```python
from build123d import *

# Parameters (mm, degrees)
F0_R     = 3.8551712717
F0_R_2   = 1.8170405965
F1_DEPTH = 12.7
F0_W     = 120.9587007761
F0_H     = 68.6061382294
F0_W_2   = 3.2722949982
F0_H_2   = 3.6340802908
F0_W_3   = 15.6750679016
F0_H_3   = 11.3066062331
F0_W_4   = 19.2726254463
F0_H_4   = 13.362351805
F2_DEPTH = 2.54


with BuildPart() as f1:
    # F0 (on Front) → F1 (new body)
    with BuildSketch(Plane.XZ):
        with BuildLine():
            Line((-130.564019084, 68.6061382294), (-120.9587007761, 68.6061382294))
            Line((-120.9587007761, 68.6061382294), (-120.9587007761, 79.2347192764))
            ThreePointArc((-120.9587007761, 79.2347192764), (-128.1642263421, 76.0919600831), (-130.564019084, 68.6061382294))
        make_face()
        with BuildLine():
            Line((120.9587007761, 79.2347192764), (120.9587007761, 68.6061382294))
            Line((120.9587007761, 68.6061382294), (130.564019084, 68.6061382294))
            ThreePointArc((130.564019084, 68.6061382294), (128.1642263421, 76.0919600831), (120.9587007761, 79.2347192764))
        make_face()
        with BuildLine():
            Line((-120.9587007761, -79.2347192764), (-120.9587007761, -68.6061382294))
            Line((-120.9587007761, -68.6061382294), (-130.564019084, -68.6061382294))
            ThreePointArc((-130.564019084, -68.6061382294), (-128.1642263421, -76.0919600831), (-120.9587007761, -79.2347192764))
        make_face()
        with BuildLine():
            Line((130.564019084, -68.6061382294), (120.9587007761, -68.6061382294))
            Line((120.9587007761, -68.6061382294), (120.9587007761, -79.2347192764))
            ThreePointArc((120.9587007761, -79.2347192764), (128.1642263421, -76.0919600831), (130.564019084, -68.6061382294))
        make_face()
        Polygon((-120.9587007761, -68.6061382294), (-120.9587007761, 0), (-120.9587007761, 68.6061382294), (-130.564019084, 68.6061382294), (-130.564019084, -68.6061382294), align=None)
        Polygon((120.9587007761, 68.6061382294), (120.9587007761, 0), (120.9587007761, -68.6061382294), (130.564019084, -68.6061382294), (130.564019084, 68.6061382294), align=None)
        Polygon((0, -68.6061382294), (-120.9587007761, -68.6061382294), (-120.9587007761, -79.2347192764), (120.9587007761, -79.2347192764), (120.9587007761, -68.6061382294), align=None)
        Polygon((-120.9587007761, 68.6061382294), (0, 68.6061382294), (120.9587007761, 68.6061382294), (120.9587007761, 79.2347192764), (-120.9587007761, 79.2347192764), align=None)
        with Locations((0, 74.081890285)):
            Circle(F0_R, mode=Mode.SUBTRACT)
        with Locations((7.9652052373, 73.8249197602)):
            Circle(F0_R_2, mode=Mode.SUBTRACT)
    extrude(amount=F1_DEPTH)

    # F0 (on Front) → F2 (join)
    with BuildSketch(Plane.XZ):
        with Locations((-60.4793503881, 34.3030691147)):
            Rectangle(F0_W, F0_H)
        with Locations((-84.6121534705, 36.4879220724)):
            Rectangle(F0_W_2, F0_H_2, mode=Mode.SUBTRACT)
        with Locations((-86.2483009696, 48.9245094359)):
            Rectangle(F0_W_3, F0_H_3, mode=Mode.SUBTRACT)
        with Locations((60.4793503881, 34.3030691147)):
            Rectangle(F0_W, F0_H)
        with Locations((71.5301930904, 45.069983229)):
            Rectangle(F0_W_4, F0_H_4, mode=Mode.SUBTRACT)
        Polygon((120.9587007761, 0), (0, 0), (0, -17.8872328252), (23.6056204885, -17.8872328252), (50.5872815847, -17.8872328252), (50.5872815847, -26.6241524369), (74.228361249, -26.6241524369), (74.228361249, -47.9525141418), (74.228361249, -55.1476255059), (62.4078214169, -55.1476255059), (62.4078214169, -47.9525141418), (50.5872815847, -47.9525141418), (50.5872815847, -44.3549603224), (20.5219965428, -44.3549603224), (0, -44.3549603224), (0, -68.6061382294), (120.9587007761, -68.6061382294), align=None)
        Polygon((0, -17.8872328252), (0, 0), (-120.9587007761, 0), (-120.9587007761, -68.6061382294), (0, -68.6061382294), (0, -44.3549603224), (-2.8621072415, -44.3549603224), (-2.8621072415, -30.9926122427), (-22.1347268671, -30.9926122427), (-22.1347268671, -28.9368666708), (-44.7479300201, -28.9368666708), (-44.7479300201, -28.6798980087), (-61.1938983202, -28.6798980087), (-61.1938983202, -40.757406503), (-77.639862895, -40.757406503), (-77.639862895, -53.0918799341), (-94.3427979946, -53.0918799341), (-111.816637218, -53.0918799341), (-111.816637218, -40.757406503), (-94.3427979946, -40.757406503), (-94.3427979946, -28.4229293466), (-77.639862895, -28.4229293466), (-77.639862895, -17.8872328252), (-61.1938983202, -17.8872328252), (-44.7479300201, -17.8872328252), (-22.1347268671, -17.8872328252), (-2.8621072415, -17.8872328252), align=None)
        with Locations((0, 74.081890285)):
            Circle(F0_R)
        with Locations((7.9652052373, 73.8249197602)):
            Circle(F0_R_2)
    extrude(amount=F2_DEPTH)


solid = f1.part
```
Geometry: final body of the model. Coordinates: model frame, mm. A direction names the side the tool comes from. Round coordinates to 2 decimals unless told otherwise and drop trailing zeros. Order: outer loops, then holes, each group sorted by start corner. A loop starts at its lowest first (then second) coordinate and runs counter-clockwise, first axis right, second up. Notation, with made-up numbers: M -7.75,-4.75 L -2.75,-4.75 A28 ccw -2.75,17.25 Z; hole C 51.5,-30 d5. An arc over 180 degrees is marked long. Use one line per item in the form item = value. Start each with the question number.
Q1. Access query for faces 1 (the face through (-2, -8, 68.606)), 2 (the face through (-1, -12.7, -70)). Directions: +Z, -Z, +X, -X, +Y, -Y. A direction counts if a zero-diameter tool reaches every point of the face in a straight line with its end or side. Return the directions, or none.
Q2. Cut plane D-D (y = -4.5). Return loops of the section in (x, z), and give its area (3 significant figures).
Q3. Cut plane A-A (x = 0). Return loops of the section in (y, z), and give its area (3 significant figures).
Q4. Cut plane B-B (z = -20.5). Return loops of the section in (x, y).
Q5. Pin query (flat end, axial travel): pin 1 Ø3 at (y, z) = (-8, -31) entering from -X; pin 2 Ø3 at (y, z) = (-1, -53) entering from +X; pin 3 Ø2 at (x, z) = (76, 4) entering from -Y. Return the tip coordinate at first contact, or that it passes through.
Q6. Mould query, pull axis Z, two halves, no side actions, for faces 3 (the face through (2, -6, 79.235)), 4 (the face through (-2, 0, 1)), 5 (the face through (-2, -6, -79.235)), 6 (the face through (120.959, -8, 1)). Classes: +Z half, -Z half, draft (parallel to the pull), parting line (faces both ways), or undercut.
Q7. Material intervals for line 1 (Z direction, x = 0, y = -8.75); line 2 (Z direction, x = 44.5, y = -9.25); line 3 (X direction, y = -7.5, z = -18), sorted ascending. Write a range as [from, to].
Q8. Cut plane C-C (z = 15). Return loops of the section in (x, y).
Geometry results:
q1.face_1 = -Y
q1.face_2 = +Z, -Z, +X, -X, -Y
q2.outline = M -130.56,-68.61 A9.54 ccw -120.96,-79.23 L 120.96,-79.23 A9.54 ccw 130.56,-68.61 L 130.56,68.61 A9.54 ccw 120.96,79.23 L -120.96,79.23 A9.54 ccw -130.56,68.61 Z; hole M -120.96,-68.61 L 120.96,-68.61 L 120.96,68.61 L -120.96,68.61 Z; hole C 0,74.08 d7.71; hole C 7.97,73.82 d3.63
q2.area = 8,050 mm^2
q3.outline = M -12.7,-79.23 L 0,-79.23 L 0,-44.35 L -2.54,-44.35 L -2.54,-68.61 L -12.7,-68.61 Z; M -12.7,68.61 L -2.54,68.61 L -2.54,-17.89 L 0,-17.89 L 0,79.23 L -12.7,79.23 L -12.7,77.94 L -2.54,77.94 L -2.54,70.23 L -12.7,70.23 Z
q3.area = 473 mm^2
q4.outline = M -130.56,-12.7 L -120.96,-12.7 L -120.96,-2.54 L -77.64,-2.54 L -77.64,0 L -130.56,0 Z; M 50.59,-2.54 L 120.96,-2.54 L 120.96,-12.7 L 130.56,-12.7 L 130.56,0 L 50.59,0 Z
q5.pin_1 = -130.56
q5.pin_2 = 130.56
q5.pin_3 = -2.54
q6.face_3 = +Z half
q6.face_4 = draft
q6.face_5 = -Z half
q6.face_6 = undercut
q7.line_1 = [-79.23, -68.61], [68.61, 70.23], [77.94, 79.23]
q7.line_2 = [-79.23, -68.61], [68.61, 79.23]
q7.line_3 = [-130.56, -120.96], [120.96, 130.56]
q8.outline = M -130.56,-12.7 L -120.96,-12.7 L -120.96,-2.54 L 120.96,-2.54 L 120.96,-12.7 L 130.56,-12.7 L 130.56,0 L -130.56,0 Z
